The listing builds one solid part. Answer for the finished solid, in the listing's coordinates (mm). Face numbers are marked on the shaded views. A direction names the side the tool comes from. Coordinates: 2 decimals unless noted, no trailing zeros. Loops run counter-clockwise (first coordinate to the right, second up) from the corner with the lowest first, then second, coordinate; pieces in that order, holes last. Notation, with made-up numbers: M -33.75,-10 L -19.75,-10 A19 cw -19.75,15 Z; hole C -20,-38 d7. An arc over 180 degrees is marked long. Answer in a Markdown table with one row per item. Add a question column.
from build123d import *

# Parameters (mm, degrees)
CROQUIS1_W              = 177.8
CROQUIS1_H              = 76.2
SALIENTE_EXTRUIR1_DEPTH = 38.1
CROQUIS2_W              = 60
CROQUIS2_H              = 60
CORTAR_EXTRUIR1_DEPTH   = 20
CROQUIS3_R              = 5
SALIENTE_EXTRUIR2_DEPTH = 15
REDONDEO1_R             = 4
REDONDEO3_R             = 4
REDONDEO4_R             = 4
REDONDEO5_R             = 4


with BuildPart() as part:
    # Croquis1 → Saliente-Extruir1 (new body)
    with BuildSketch(Plane.XY):
        Rectangle(CROQUIS1_W, CROQUIS1_H)
    extrude(amount=SALIENTE_EXTRUIR1_DEPTH)

    # Croquis2 → Cortar-Extruir1 (cut)
    with BuildSketch(Plane.XY.offset(38.1)):
        with Locations((44.45, 0)):
            Rectangle(CROQUIS2_W, CROQUIS2_H)
    extrude(amount=-CORTAR_EXTRUIR1_DEPTH, mode=Mode.SUBTRACT)

    # Croquis3 → Saliente-Extruir2 (add)
    with BuildSketch(Plane.XY.offset(18.1)):
        Polygon((44.45, 23.094010768), (24.45, 11.547005384), (24.45, -11.547005384), (44.45, -23.094010768), (64.45, -11.547005384), (64.45, 11.547005384), align=None)
        with Locations((44.45, 0)):
            Circle(CROQUIS3_R, mode=Mode.SUBTRACT)
    extrude(amount=SALIENTE_EXTRUIR2_DEPTH)

    # Redondeo1
    redondeo1_edges = [part.edges().sort_by_distance(p)[0] for p in [
        (14.45, 0, 18.1),
        (14.45, -30, 28.1),
        (44.45, 30, 18.1),
        (14.45, 30, 28.1),
        (74.45, 0, 18.1),
        (74.45, 30, 28.1),
        (44.45, -30, 18.1),
        (74.45, -30, 28.1),
    ]]
    fillet(redondeo1_edges, radius=REDONDEO1_R)

    # Redondeo3
    redondeo3_edges = [part.edges().sort_by_distance(p)[0] for p in [
        (64.45, 11.547005384, 25.6),
        (44.45, 23.094010768, 25.6),
        (24.45, 11.547005384, 25.6),
        (24.45, -11.547005384, 25.6),
        (44.45, -23.094010768, 25.6),
        (64.45, -11.547005384, 25.6),
    ]]
    fillet(redondeo3_edges, radius=REDONDEO3_R)

    # Redondeo4
    redondeo4_edges = [part.edges().sort_by_distance(p)[0] for p in [
        (39.45, 0, 33.1),
    ]]
    fillet(redondeo4_edges, radius=REDONDEO4_R)

    # Redondeo5
    redondeo5_edges = [part.edges().sort_by_distance(p)[0] for p in [
        (44.45, 22.475208614, 33.1),
        (24.985898385, 11.237604307, 33.1),
        (24.985898385, -11.237604307, 33.1),
        (44.45, -22.475208614, 33.1),
        (63.914101615, -11.237604307, 33.1),
        (63.914101615, 11.237604307, 33.1),
        (54.45, 17.320508076, 33.1),
        (64.45, 0, 33.1),
        (34.45, 17.320508076, 33.1),
        (24.45, 0, 33.1),
        (34.45, -17.320508076, 33.1),
        (54.45, -17.320508076, 33.1),
    ]]
    fillet(redondeo5_edges, radius=REDONDEO5_R)


solid = part.part
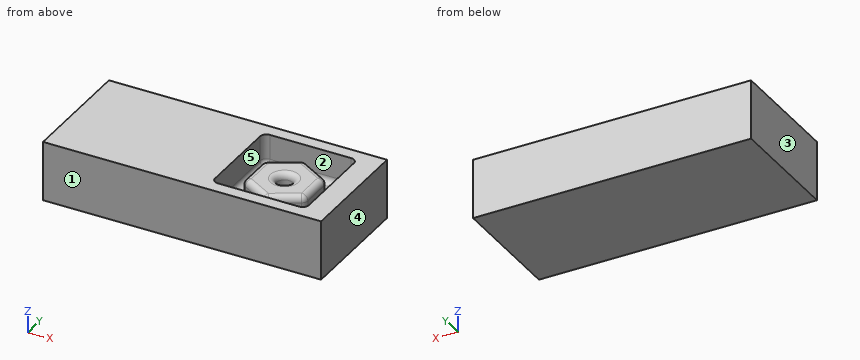
(1) Each of these flat-tipped pins is pushed along its axis until it touches: pin 1 (11 mm diameter, centred on x = 45, y = 1.5, fed in from +Z); pin 2 (1.5 mm diameter, centred on x = -37.5, y = 17, fed in from -Z); pin 3 (13 mm diameter, centred on x = 44.45, y = 0, fed in from +Z); pin 4 (16 mm diameter, centred on x = 46, y = -1.5, fed in from +Z). Where does it stop, or does it pass through?
(2) Straight lines are drawn through the part: line 1 (Y direction, x = 44.45, z = 23); line 2 (Y direction, x = 44, z = 24); line 3 (Y direction, x = 36, z = 32). For each, find the intervals that lie inside material, in ascending order.
(3) The mould has two halves that part along X. Classify the marked faces 1, 2 and 3: released by +X, released by -X, zero draft, split by the parting line, or undercut.
(4) A cutting plane is placed at A-A (z = 27). Give the vertices of the cut face in (x, y), plus the area to 3 significant figures.
(5) A cutting plane is placed at B-B (y = 0). Give the vertices of the cut face in (x, z), plus the area to 3 significant figures.
(6) For the marked faces 4 and 5, determine the directions among +Z, -Z, +X, -X, +Y, -Y from which every point of the face is accessible in a straight line to the end or side of a thin tool.
Solved:
| question | item | result |
|---|---|---|
| 1 | pin 1 | stops at z = 32.62 |
| 1 | pin 2 | stops at z = 0 |
| 1 | pin 3 | stops at z = 32.22 |
| 1 | pin 4 | stops at z = 33.1 |
| 2 | line 1 | y = -38.1 to -30, -22.48 to -5, 5 to 22.48, 30 to 38.1 |
| 2 | line 2 | y = -38.1 to -30, -22.45 to -4.98, 4.98 to 22.45, 30 to 38.1 |
| 2 | line 3 | y = -38.1 to -30, -16.78 to 16.78, 30 to 38.1 |
| 3 | face 1 | zero draft |
| 3 | face 2 | undercut |
| 3 | face 3 | released by -X |
| 4 | outline | M -88.9,-38.1 L 88.9,-38.1 L 88.9,38.1 L -88.9,38.1 Z; M 24.45,-9.24 A4 ccw 26.45,-12.7 L 42.45,-21.94 A4 ccw 46.45,-21.94 L 62.45,-12.7 A4 ccw 64.45,-9.24 L 64.45,9.24 A4 ccw 62.45,12.7 L 46.45,21.94 A4 ccw 42.45,21.94 L 26.45,12.7 A4 ccw 24.45,9.24 Z; hole M 14.45,-26 A4 ccw 18.45,-30 L 70.45,-30 A4 ccw 74.45,-26 L 74.45,26 A4 ccw 70.45,30 L 18.45,30 A4 ccw 14.45,26 Z; hole C 44.45,0 d10 |
| 4 | area | 11,300 mm² |
| 5 | outline | M -88.9,0 L 88.9,0 L 88.9,38.1 L 74.45,38.1 L 74.45,22.1 A4 cw 70.45,18.1 L 64.45,18.1 L 64.45,29.1 A4 ccw 60.45,33.1 L 53.45,33.1 A4 ccw 49.45,29.1 L 49.45,18.1 L 39.45,18.1 L 39.45,29.1 A4 ccw 35.45,33.1 L 28.45,33.1 A4 ccw 24.45,29.1 L 24.45,18.1 L 18.45,18.1 A4 cw 14.45,22.1 L 14.45,38.1 L -88.9,38.1 Z |
| 5 | area | 6,020 mm² |
| 6 | face 4 | +Z, -Z, +X, +Y, -Y |
| 6 | face 5 | +Z |
